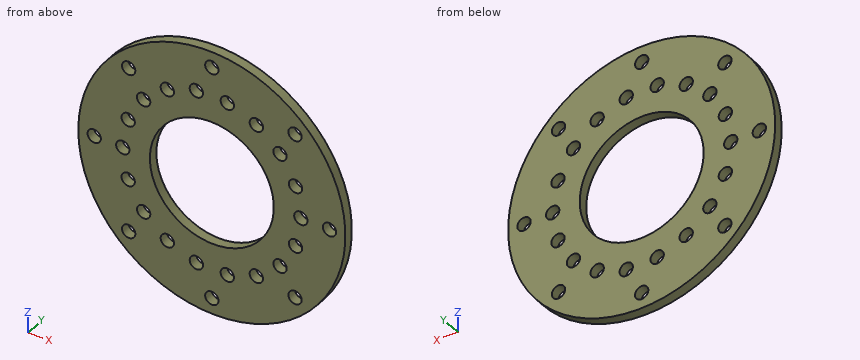
Autodesk Inventor part; units mm, degrees
ref_plane "YZ Plane" through (0, 0, 0) normal (1, 0, 0) x (0, 1, 0)
ref_plane "XZ Plane" through (0, 0, 0) normal (0, 1, 0) x (-1, 0, 0)
ref_plane "XY Plane" through (0, 0, 0) normal (0, 0, 1) x (1, 0, 0)
sketch "Sketch1" plane through (0, 0, 0) normal (0, 1, 0) x (-1, 0, 0)
  circle A0 centre (0, 0) radius 42
  circle A1 centre (0, 0) radius 19.5
  circle A2 centre (0, -37) radius 2.1
  circle A3 centre (26.163, -26.163) radius 2.1
  circle A4 centre (37, 0) radius 2.1
  circle A5 centre (26.163, 26.163) radius 2.1
  circle A6 centre (0, 37) radius 2.1
  circle A7 centre (-26.163, 26.163) radius 2.1
  circle A8 centre (-37, 0) radius 2.1
  circle A9 centre (-26.163, -26.163) radius 2.1
  circle A10 centre (-4.8621, -27.5746) radius 2.1
  circle A11 centre (4.8621, -27.5746) radius 2.1
  circle A12 centre (14, -24.2487) radius 2.1
  circle A13 centre (21.4492, -17.9981) radius 2.1
  circle A14 centre (26.3114, -9.5766) radius 2.1
  circle A15 centre (28, 0) radius 2.1
  circle A16 centre (26.3114, 9.5766) radius 2.1
  circle A17 centre (21.4492, 17.9981) radius 2.1
  circle A18 centre (14, 24.2487) radius 2.1
  circle A19 centre (4.8621, 27.5746) radius 2.1
  circle A20 centre (-4.8621, 27.5746) radius 2.1
  circle A21 centre (-14, 24.2487) radius 2.1
  circle A22 centre (-21.4492, 17.9981) radius 2.1
  circle A23 centre (-26.3114, 9.5766) radius 2.1
  circle A24 centre (-28, 0) radius 2.1
  circle A25 centre (-26.3114, -9.5766) radius 2.1
  circle A26 centre (-21.4492, -17.9981) radius 2.1
  circle A27 centre (-14, -24.2487) radius 2.1
  line L0 (0, 0) -> (-4.8621, -27.5746) construction
  line L1 (0, 0) -> (0, -11.0753) construction
  dimension "d2" = 84
  dimension "d3" = 39
  dimension "d4" = 4.2
  dimension "d5" = 37
  dimension "d6" = 360
  dimension "d9" = 4.2
  dimension "d10" = 28
  dimension "d11" = 360
  dimension "d12" = 10
extrude "Extrusion1" add sketch "Sketch1" along normal blind 3
properties part number "NewHousingLid"
Check sheet for the modelled part. Datum: model origin and axes. Units: mm. Round coordinates to 2 decimals unless told otherwise and drop trailing zeros. Order: outer loops, then holes, each group sorted by start corner. A loop starts at its lowest first (then second) coordinate and runs counter-clockwise, first axis right, second up.
Q1. Depth check by flat-ended pin: P1, Ø1.5, axis at y = 1, z = -17, coming from the -X side; P2, Ø1, axis at x = 9, y = 1.5, coming from the -Z side. Enter the tip coordinate at first touch or a pass-through.
Filled sheet:
P1: stops at x = -38.73
P2: stops at z = -41.13
Q2. Scan lines: L1, parallel to Z at x = 5.5, y = 1.7; L2, parallel to X at y = 2.7, z = 1.5; L3, parallel to X at y = 0.15, z = -28.5. Record each from-to range of solid material in increasing order.
Filled sheet:
L1: z = -41.64 to -29.58, -25.57 to -18.71, 18.71 to 25.57, 29.58 to 41.64
L2: x = -41.97 to -38.47, -35.53 to -29.47, -26.53 to -19.44, 19.44 to 26.53, 29.47 to 35.53, 38.47 to 41.97
L3: x = -30.85 to -6.75, -2.98 to 2.98, 6.75 to 30.85
Q3. Cross-section at D-D, the plane x = -21. Enter the section's corners in (y, z).
Filled sheet:
outline: (0, -36.37) - (3, -36.37) - (3, -20.05) - (0, -20.05) - close; (0, -15.95) - (3, -15.95) - (3, 15.95) - (0, 15.95) - close; (0, 20.05) - (3, 20.05) - (3, 36.37) - (0, 36.37) - close
Q4. Cross-section at C-C, the plane z = -37. Enter the section's corners in (x, y), plus the area to 3 significant figures.
Filled sheet:
outline: (-19.87, 0) - (-2.1, 0) - (-2.1, 3) - (-19.87, 3) - close; (2.1, 0) - (19.87, 0) - (19.87, 3) - (2.1, 3) - close
area: 107 mm2
Q5. Cross-section at A-A, the plane x = 0. Enter the section's corners in (y, z).
Filled sheet:
outline: (0, -42) - (3, -42) - (3, -39.1) - (0, -39.1) - close; (0, -34.9) - (3, -34.9) - (3, -19.5) - (0, -19.5) - close; (0, 19.5) - (3, 19.5) - (3, 34.9) - (0, 34.9) - close; (0, 39.1) - (3, 39.1) - (3, 42) - (0, 42) - close
Q6. Cross-section at B-B, the plane y = 0.9. Give the number of separate pieces and of enclosed holes in the cut face, plus the area to 3 significant figures.
Filled sheet:
separate pieces: 1
enclosed holes: 27
area: 3,990 mm2
